```python
from build123d import *

# Parameters (mm, degrees)
SKETCH1_R                  = 42.5
SKETCH1_R_2                = 35
BOSS_EXTRUDE1_DEPTH        = 110
BOSS_EXTRUDE2_REACH        = 187.35
BOSS_EXTRUDE2_START_RADIUS = 42.5
BOSS_EXTRUDE2_END_RADIUS   = 42.5
SKETCH2_W                  = 5
SKETCH2_H                  = 105


with BuildPart() as part:
    # Sketch1 → Boss-Extrude1 (new body)
    with BuildSketch(Plane(origin=(0, 0, 0), x_dir=(1, 0, 0), z_dir=(0, 1, 0))):
        with Locations(Location((0, 0, 0), (0, 0, 270))):
            Circle(SKETCH1_R)
        with Locations(Location((0, 0, 0), (0, 0, 270))):
            Circle(SKETCH1_R_2, mode=Mode.SUBTRACT)
    extrude(amount=BOSS_EXTRUDE1_DEPTH)

    # Boss-Extrude2: from a cylinder face, 187.35 long prism both ways, kept between that surface and its translate by the depth
    boss_extrude2_start = Plane(origin=(0, 55, 0), z_dir=(0, -1, 0)) * Cylinder(BOSS_EXTRUDE2_START_RADIUS, 460.7, mode=Mode.PRIVATE)
    boss_extrude2_end = Plane(origin=(60, 55, 0), z_dir=(0, -1, 0)) * Cylinder(BOSS_EXTRUDE2_END_RADIUS, 460.7, mode=Mode.PRIVATE)
    # Sketch2 → Boss-Extrude2 (add, from a surface)
    with BuildSketch(Plane(origin=(0, 0, 0), x_dir=(0, 0, -1), z_dir=(1, 0, 0)), mode=Mode.PRIVATE) as boss_extrude2_sk1:
        with Locations((0, 55)):
            Rectangle(SKETCH2_W, SKETCH2_H)
    boss_extrude2_tool1 = extrude(boss_extrude2_sk1.sketch, amount=BOSS_EXTRUDE2_REACH, both=True, mode=Mode.PRIVATE)
    add(((boss_extrude2_tool1 - boss_extrude2_start) & boss_extrude2_end).solids().sort_by_distance((72.426407, 55, 0))[0])


solid = part.part
```
Design review of the part built by this model. Coordinates are the model's own, in mm. A direction names the side the tool comes from. Give positions to 0.01 mm unless a question says otherwise; leave off trailing zeros. Order: outer loops, then holes, each group sorted by start corner. A loop starts at its lowest first (then second) coordinate and runs counter-clockwise, first axis right, second up. Notation, with made-up numbers: (9.5, 84.25) -> (15.5, 84.25) arc R28 cw to (15.5, 103.25) -> close; hole circle Ø5 at (54, 74.25). An arc over 180 degrees is marked (long way). Write each question's results on one line, items separated by ' | '. Start each with the question number.
Q1. Wall thickness on L1, parallel to X at y = 44, z = 0; L2, parallel to X at y = 73, z = 16; L3, parallel to Z at x = -8, y = 56.5: over which ranges is each line inside the solid? List them lowest first. Write a range as from..to.
Q2. For pin 1 (2.5 mm diameter, centred on x = 86.5, z = 0, fed in from -Y); pin 2 (2 mm diameter, centred on x = 2, y = 67, fed in from -Z); pin 3 (12 mm diameter, centred on y = 64.5, z = -13.5, fed in from -X); pin 4 (2 mm diameter, centred on x = 44.5, z = 4.5, fed in from -Y), all flat-tipped, find the tip position at first contact; note any pin that passes through.
Q3. Add section B-B on x = 0. Give the boundary of the cut face in (y, z), and give its area (3 significant figures).
Q4. Mouldability with a two-part tool opening along X and no side actions: class faces 1 (the cylindrical face through (102.5, 54.3, 0)), 2 (the cylindrical face through (-21, 54, -28)), 3 (the flat face through (73, 54, 2.5)), 4 (the cylindrical face through (-25.861, 54.23, -33.727)) as +X half, -X half, draft (parallel to the pull), parting line (faces both ways), or undercut.
Q5. Add section D-D on x = -26. Give the boundary of the cut face in (y, z), and give its area (3 significant figures).
Q6. Machinability: for faces 5 (the flat face through (35, 110, 6)), 6 (the flat face through (73, 107.5, 0)), 7 (the flat face through (73, 2.5, 0)), 8 (the flat face through (73, 54, -2.5)), which of the approach directions +Z, -Z, +X, -X, +Y, -Y give a long, thin tool a straight path to every point of the face, cutting with its end or side? Answer none if there is none.
Q7. Add section C-C on y = 44.5. Give the boundary of the cut face in (x, z).
Q8. Add section A-A on z = 0. Give the boundary of the cut face in (x, y), and give its area (3 significant figures).
Found:
1) L1: x = -42.5..-35, 35..102.5 | L2: x = -39.37..-31.13, 31.13..39.37 | L3: z = -41.74..-34.07, 34.07..41.74
2) pin 1: stops at y = 2.5 | pin 2: stops at z = -42.49 | pin 3: stops at x = -41.83 | pin 4: passes through
3) outline: (0, -42.5) -> (110, -42.5) -> (110, -35) -> (0, -35) -> close; (0, 35) -> (110, 35) -> (110, 42.5) -> (0, 42.5) -> close | area: 1,650 mm2
4) face 1: +X half | face 2: undercut | face 3: draft | face 4: parting line
5) outline: (0, -33.62) -> (110, -33.62) -> (110, -23.43) -> (0, -23.43) -> close; (0, 23.43) -> (110, 23.43) -> (110, 33.62) -> (0, 33.62) -> close | area: 2,240 mm2
6) face 5: +Z, -Z, +X, -X, +Y | face 6: +Z, -Z, +X, +Y | face 7: +Z, -Z, +X, -Y | face 8: -Z, +X, +Y, -Y
7) outline: (42.43, -2.5) -> (102.43, -2.5) arc R42.5 ccw to (102.43, 2.5) -> (42.43, 2.5) arc R42.5 ccw (long way) to start; hole circle Ø70 at (0, 0)
8) outline: (-42.5, 0) -> (-35, 0) -> (-35, 110) -> (-42.5, 110) -> close; (35, 0) -> (42.5, 0) -> (42.5, 2.5) -> (102.5, 2.5) -> (102.5, 107.5) -> (42.5, 107.5) -> (42.5, 110) -> (35, 110) -> close | area: 7,950 mm2
